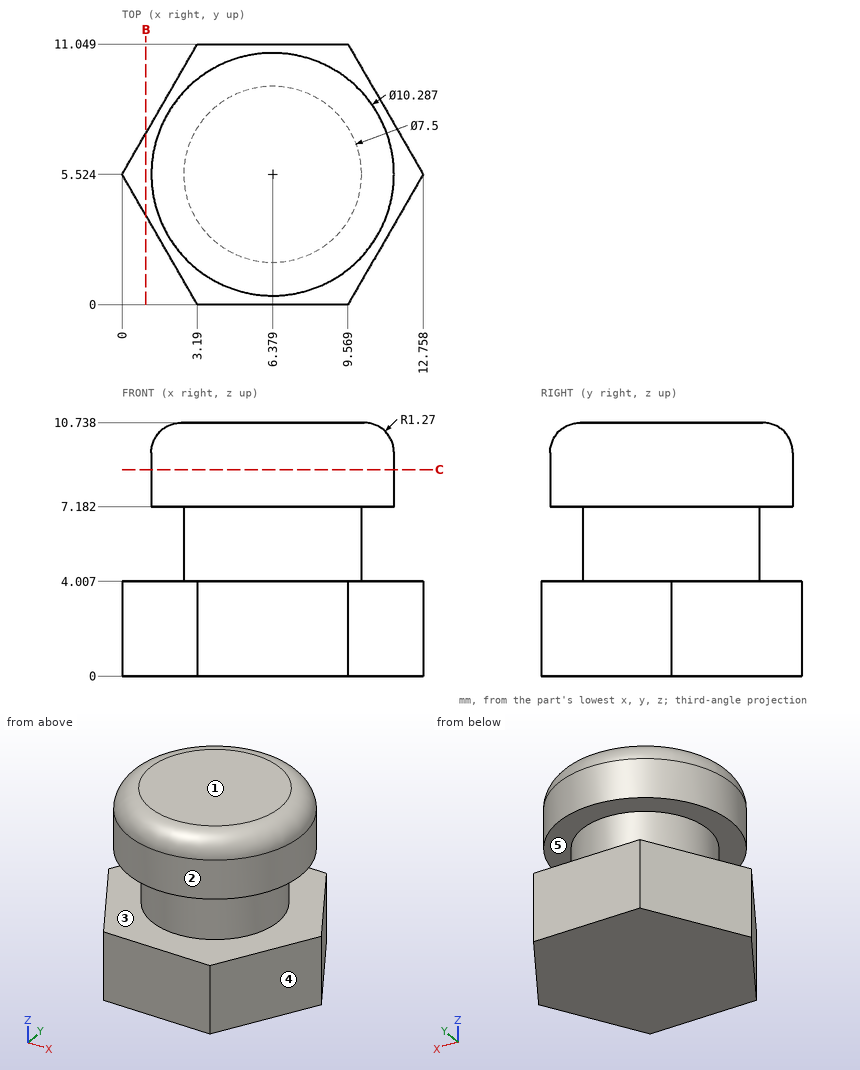
The figure shows three views and two pictorial views of one solid part (mm, origin at its lowest corner). Answer the questions. A direction names the side the tool comes from. Round coordinates to 2 decimals unless told otherwise and drop trailing zeros. Order: outer loops, then holes, each group sorted by start corner. A loop starts at its lowest first (then second) coordinate and runs counter-clockwise, first axis right, second up. Notation, with made-up numbers: M 49.5,52 L 57.5,52 A18 cw 57.5,71 Z; hole C 70,72 d6. An arc over 180 degrees is marked long. Answer in a Markdown table with one row per item. Add a question column.
1) Determine the mould class of the marked faces 1, 2 and 3 for opening direction Z: pulls with the +Z half, pulls with the -Z half, needs draft (parallel to the pull), parting line crosses it, or undercut.
2) The part is cut by section B-B on x = 1. Determine the outline of the cut face in (y, z), plus the area to 3 significant figures.
3) Flat-ended cylindrical pins translate along their axes: pin 1 Ø1 at (x, z) = (8, 1) entering from -Y; pin 2 Ø4 at (x, z) = (8.5, 7.5) entering from -Y; pin 3 Ø1.5 at (y, z) = (2, 4.5) entering from -X. Find the tip coordinate at first contact, or state that the pin passes through.
4) The part is cut by section C-C on z = 8.75. Determine the outline of the cut face in (x, y) (1 decimal).
5) Consider line 1 along Z through (x, y) = (12, 5.5); line 2 along Z through (x, y) = (10.75, 3.75) (1 decimal); line 3 along Y through (x, z) = (3, 7.75) (1 decimal). Determine where each line is inside the solid, lowest interval first. Write a range as from..to.
6) Which of the six approach directions +Z, -Z, +X, -X, +Y, -Y give full straight-line access (tool end or side, diameter ignored) to the marked faces 4 and 5?
Findings below:
| question | item | result |
|---|---|---|
| 1 | face 1 | pulls with the +Z half |
| 1 | face 2 | needs draft |
| 1 | face 3 | undercut |
| 2 | outline | M 3.79,0 L 7.26,0 L 7.26,4.01 L 3.79,4.01 Z |
| 2 | area | 13.9 mm² |
| 3 | pin 1 | stops at y = 0 |
| 3 | pin 2 | stops at y = 0.38 |
| 3 | pin 3 | stops at x = 1.71 |
| 4 | outline | C 6.4,5.5 d10.3 |
| 5 | line 1 | z = 0..4.01 |
| 5 | line 2 | z = 0..4, 7.2..10.4 |
| 5 | line 3 | y = 1.6..9.4 |
| 6 | face 4 | +Z, -Z, +X, -Y |
| 6 | face 5 | none |
